Can you work these out from the model? Positions are in its coordinate system, mm. Coordinates: 2 decimals unless noted, no trailing zeros. Loops run counter-clockwise (first coordinate to the right, second up) from the corner with the lowest first, then second, coordinate; pieces in that order, holes last.
```python
from build123d import *

# Parameters (mm, degrees)
PAD013_DEPTH            = 12
CHAMFER013_SIZE         = 6.9
FILLET028_R             = 1
FILLET027_R             = 3
FILLET029_R             = 1
SKETCH052_R             = 1.25
POCKET020_DEPTH         = 109.001
CHAMFER014_SIZE         = 0.5
FILLET031_R             = 1
BODY012_PLACEMENT_ANGLE = 180


with BuildPart() as part:
    # Sketch051 → Pad013 (new body)
    with BuildSketch(Plane.YZ.offset(37)):
        Polygon((-48, 6), (-41, 6), (-41, 13), (54, 13), (54, 6), (61, 6), (61, 22), (-48, 22), align=None)
    extrude(amount=PAD013_DEPTH)

    # Chamfer013
    chamfer013_edges = [part.edges().sort_by_distance(p)[0] for p in [
        (49, 6.5, 22),
    ]]
    chamfer(chamfer013_edges, length=CHAMFER013_SIZE)

    # Fillet028
    fillet028_edges = [part.edges().sort_by_distance(p)[0] for p in [
        (49, 6.5, 13),
    ]]
    fillet(fillet028_edges, radius=FILLET028_R)

    # Fillet027
    fillet027_edges = [part.edges().sort_by_distance(p)[0] for p in [
        (49, 57.5, 6),
        (49, -44.5, 6),
    ]]
    fillet(fillet027_edges, radius=FILLET027_R)

    # Fillet029
    fillet029_edges = [part.edges().sort_by_distance(p)[0] for p in [
        (41.5, 61, 6),
        (48.12132, 61, 6.87868),
        (49, 61, 12.05),
        (45.55, 61, 18.55),
        (39.55, 61, 22),
    ]]
    fillet(fillet029_edges, radius=FILLET029_R)

    # Sketch052 (on Face12 of Fillet029) → Pocket020 (cut, through all)
    with BuildSketch(Plane.ZX.offset(61)):
        with Locations((9.54001, 44.356239)):
            Circle(SKETCH052_R)
    extrude(amount=-POCKET020_DEPTH, mode=Mode.SUBTRACT)

    # Chamfer014
    chamfer014_edges = [part.edges().sort_by_distance(p)[0] for p in [
        (44.356239, 61, 8.29001),
        (44.356239, -48, 8.29001),
    ]]
    chamfer(chamfer014_edges, length=CHAMFER014_SIZE)

    # Fillet031
    fillet031_edges = [part.edges().sort_by_distance(p)[0] for p in [
        (41.5, -48, 6),
        (48.12132, -48, 6.87868),
        (49, -48, 12.05),
        (45.55, -48, 18.55),
        (39.55, -48, 22),
    ]]
    fillet(fillet031_edges, radius=FILLET031_R)


with BuildPart() as part_1:
    # Body012 placement: moved
    add(part.part.moved(Location((7.57, 12.98, 9.09))).rotate(Axis((7.57, 12.98, 9.09), (1, 0, 0)), BODY012_PLACEMENT_ANGLE))


solid = part_1.part
```
Item 1: Suppose I cut it at B-B, the plane y = -37. Please give me the cut outline in (x, z), plus the area to 3 significant figures.
Results are:
outline: (44.57, -12.91) - (49.67, -12.91) - (56.57, -6.01) - (56.57, -4.91) arc R1 ccw to (55.57, -3.91) - (44.57, -3.91) - close
area: 84.0 mm2
Item 2: We'd pull the mould along Y, two halves only. Please class faces 1 (the face through (49, 60.98, -5)), 2 (the face through (49, 57, 3.09)), 3 (the face through (50, 7, -3.91)): +Y half, -Y half, draft (parallel to the pull), parting line (faces both ways), or undercut.
Results are:
face 1: +Y half
face 2: draft
face 3: undercut
Item 3: I'm going to push flat-ended pins straight in: P1, Ø2, axis at x = 48, y = 29.5, coming from the +Z side; P2, Ø1.5, axis at x = 51.93, z = -0.45, coming from the -Y side. Where does each tip first touch, or does it pass through?
Results are:
P1: stops at z = -3.91
P2: passes through
Item 4: Suppose I cut it at A-A, the plane x = 47.5. Please give me the cut outline in (y, z), plus the area to 3 significant figures.
Results are:
outline: (-48.02, -11.91) arc R1 ccw to (-47.02, -12.91) - (59.98, -12.91) arc R1 ccw to (60.98, -11.91) - (60.98, 2.09) arc R1 ccw to (59.98, 3.09) - (53.98, 3.09) - (53.98, -3.91) - (-41.02, -3.91) - (-41.02, 3.09) - (-47.02, 3.09) arc R1 ccw to (-48.02, 2.09) - close
area: 1,080 mm2
Item 5: I need wall thicknesses on line 1 along Y through (x, z) = (53.5, -1.75); line 2 along Z through (x, y) = (45.5, 7); line 3 along Y through (x, z) = (51, 0.5). Which ranges of each line are inside material? Lowest first, please.
Results are:
line 1: y = -48.02 to -41.02, 53.98 to 60.98
line 2: z = -12.91 to -3.91
line 3: y = -47.6 to -41.02, 53.98 to 60.56
